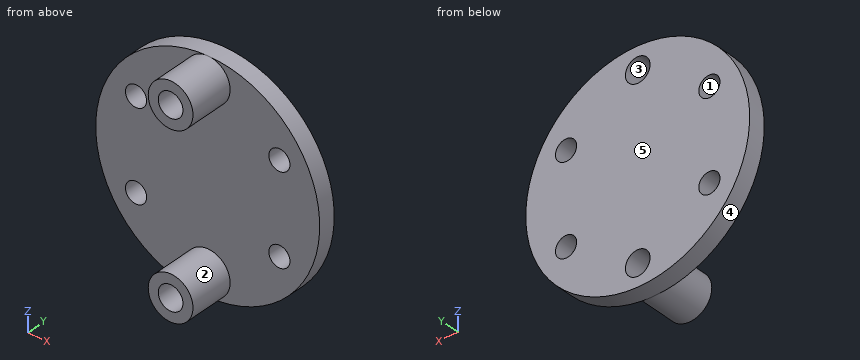
```python
from build123d import *

# Parameters (mm, degrees)
SKETCH1_R           = 15.875
SKETCH1_R_2         = 1.5
SKETCH1_R_3         = 1.75
BOSS_EXTRUDE1_DEPTH = 2.54
BOSS_EXTRUDE2_START = -6.474999999
SKETCH1_3_R         = 3.175
SKETCH1_3_R_2       = 1.75
BOSS_EXTRUDE2_DEPTH = 6.474999999


with BuildPart() as part:
    # Sketch1 → Boss-Extrude1 (new body)
    with BuildSketch(Plane(origin=(0, 0, 0), x_dir=(1, 0, 0), z_dir=(0, 1, 0))):
        with Locations(Location((0, 0, 0), (0, 0, 270))):
            Circle(SKETCH1_R)
        with Locations(Location((-10.16, 6.35, 0), (0, 0, 270))):
            Circle(SKETCH1_R_2, mode=Mode.SUBTRACT)
        with Locations(Location((10.16, 6.35, 0), (0, 0, 270))):
            Circle(SKETCH1_R_2, mode=Mode.SUBTRACT)
        with Locations(Location((10.16, -6.35, 0), (0, 0, 270))):
            Circle(SKETCH1_R_2, mode=Mode.SUBTRACT)
        with Locations(Location((-10.16, -6.35, 0), (0, 0, 270))):
            Circle(SKETCH1_R_2, mode=Mode.SUBTRACT)
        with Locations(Location((0, 12.7, 0), (0, 0, 270))):
            Circle(SKETCH1_R_3, mode=Mode.SUBTRACT)
        with Locations(Location((0, -12.7, 0), (0, 0, 270))):
            Circle(SKETCH1_R_3, mode=Mode.SUBTRACT)
    extrude(amount=BOSS_EXTRUDE1_DEPTH)

    # Sketch1_3 → Boss-Extrude2 (add)
    # profile 1 of 2: a face of its own
    with BuildSketch(Plane(origin=(0, 0, 0), x_dir=(1, 0, 0), z_dir=(0, 1, 0)).offset(BOSS_EXTRUDE2_START)):
        with Locations(Location((0, 12.7, 0), (0, 0, 270))):
            Circle(SKETCH1_3_R)
        with Locations(Location((0, 12.7, 0), (0, 0, 270))):
            Circle(SKETCH1_3_R_2, mode=Mode.SUBTRACT)
    # profile 2 of 2: a face of its own
    with BuildSketch(Plane(origin=(0, 0, 0), x_dir=(1, 0, 0), z_dir=(0, 1, 0)).offset(BOSS_EXTRUDE2_START)):
        with Locations(Location((0, -12.7, 0), (0, 0, 270))):
            Circle(SKETCH1_3_R)
        with Locations(Location((0, -12.7, 0), (0, 0, 270))):
            Circle(SKETCH1_3_R_2, mode=Mode.SUBTRACT)
    extrude(amount=BOSS_EXTRUDE2_DEPTH)


solid = part.part
```
Source: CAD feature listing. Evaluate the final solid. Frame: model axes, mm. Face numbers are marked on the shaded views. A direction names the side the tool comes from. Round coordinates to 2 decimals unless told otherwise and drop trailing zeros. Order: outer loops, then holes, each group sorted by start corner. A loop starts at its lowest first (then second) coordinate and runs counter-clockwise, first axis right, second up. Notation, with made-up numbers: (41.5, 64) -> (95.5, 64) arc R14 cw to (95.5, 70) -> close; hole circle Ø10 at (76.25, 26). An arc over 180 degrees is marked (long way). One line per item, written item: value. Start each with the question number.
Q1. Draft query along Z for the marked faces 3, 4 and 5. Return one class per face: pulls with the +Z half, pulls with the -Z half, needs draft (parallel to the pull), parting line crosses it, or undercut.
Q2. Access query for the marked faces 1 and 2. Directions: +Z, -Z, +X, -X, +Y, -Y. A direction counts if a zero-diameter tool reaches every point of the face in a straight line with its end or side. Return the directions, or none.
Q3. Section query D-D (z = -5.5). Return the cut outline in (x, y), plus the area to 3 significant figures.
Q4. Section query B-B (z = 12.7). Return the cut outline in (x, y) (3 decimals), plus the area to 3 significant figures.
Q5. Material intervals for probe 1 along X at (y, z) = (1.85, 6.35); probe 2 along X at (y, z) = (-1.5, 12.7) (3 decimals); probe 3 along X at (y, z) = (1.25, 6), sorted ascending.
Q6. Section query C-C (x = 10.16). Return the cut outline in (y, z), plus the area to 3 significant figures.
Q7. Pin query (flat end, axial travel): pin 1 (5 mm diameter, centred on x = 5, z = 2.5, fed in from -Y); pin 2 (3 mm diameter, centred on x = 6, y = -4.5, fed in from +Z). Return the tip coordinate at first contact, or that it passes through.
Q8. Section query A-A (y = 1.5). Return the cut outline in (x, z) (3 decimals), plus the area to 3 significant figures.
Findings below:
1. face 3: undercut
1. face 4: parting line crosses it
1. face 5: needs draft
2. face 1: +Y, -Y
2. face 2: -Y
3. outline: (-14.89, 0) -> (-11.4, 0) -> (-11.4, 2.54) -> (-14.89, 2.54) -> close; (-8.92, 0) -> (8.92, 0) -> (8.92, 2.54) -> (-8.92, 2.54) -> close; (11.4, 0) -> (14.89, 0) -> (14.89, 2.54) -> (11.4, 2.54) -> close
3. area: 63.1 mm²
4. outline: (-9.525, 0) -> (-3.175, 0) -> (-3.175, -6.475) -> (-1.75, -6.475) -> (-1.75, 2.54) -> (-9.525, 2.54) -> close; (1.75, -6.475) -> (3.175, -6.475) -> (3.175, 0) -> (9.525, 0) -> (9.525, 2.54) -> (1.75, 2.54) -> close
4. area: 58.0 mm²
5. probe 1: -14.55 to -11.66, -8.66 to 8.66, 11.66 to 14.55
5. probe 2: -3.175 to -1.75, 1.75 to 3.175
5. probe 3: -14.7 to -11.62, -8.7 to 8.7, 11.62 to 14.7
6. outline: (0, -12.2) -> (2.54, -12.2) -> (2.54, -7.85) -> (0, -7.85) -> close; (0, -4.85) -> (2.54, -4.85) -> (2.54, 4.85) -> (0, 4.85) -> close; (0, 7.85) -> (2.54, 7.85) -> (2.54, 12.2) -> (0, 12.2) -> close
6. area: 46.7 mm²
7. pin 1: y = 0
7. pin 2: through
8. outline: circle Ø31.75 at (0, 0); hole circle Ø3 at (-10.16, -6.35); hole circle Ø3 at (-10.16, 6.35); hole circle Ø3.5 at (0, -12.7); hole circle Ø3.5 at (0, 12.7); hole circle Ø3 at (10.16, -6.35); hole circle Ø3 at (10.16, 6.35)
8. area: 744 mm²
